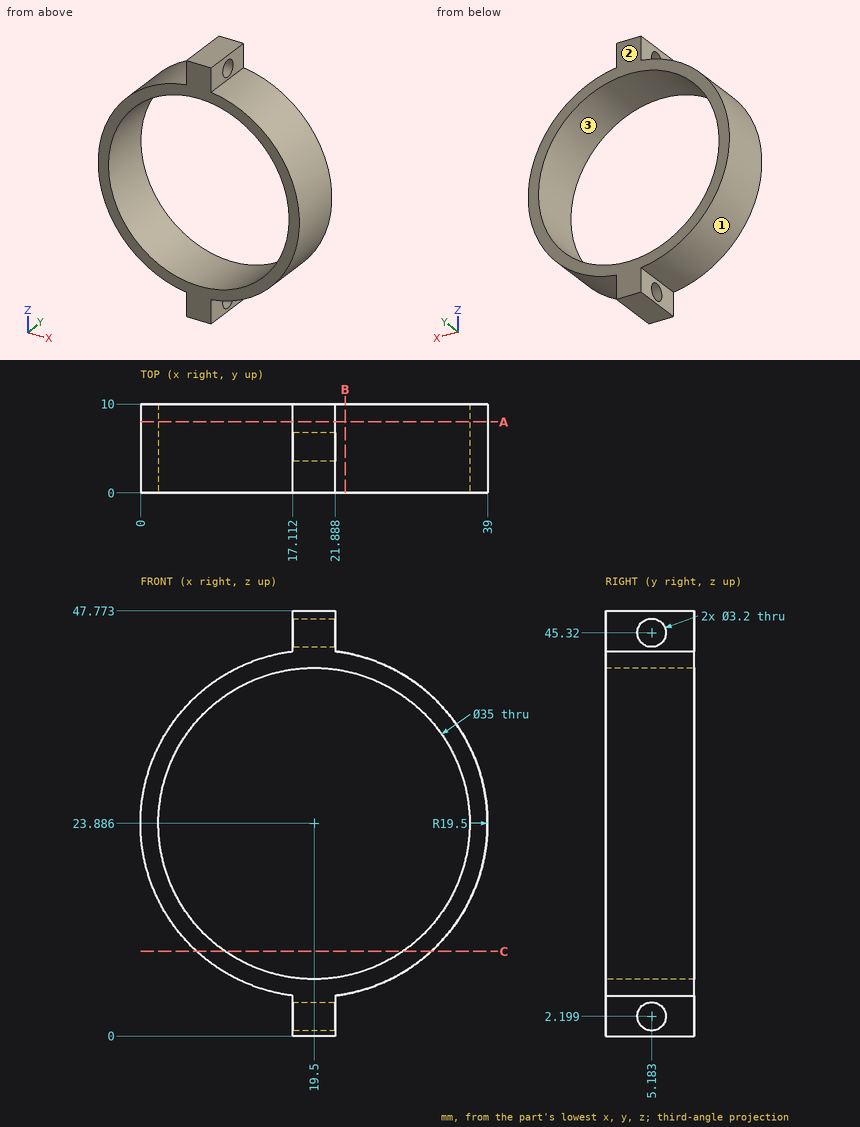
For this review, use the dimensioned drawing (mm, ordinates from the lowest corner) and the shaded views. Give positions to 0.01 mm unless a question says otherwise; leave off trailing zeros. Order: outer loops, then holes, each group sorted by start corner. A loop starts at its lowest first (then second) coordinate and runs counter-clockwise, first axis right, second up. Notation, with made-up numbers: (-21, 42) - (13, 42) arc R21 ccw to (13, 78) - close; hole circle Ø9 at (47, 65). An arc over 180 degrees is marked (long way). Write item = value, one per line. Start each with the question number.
Q1. We need section B-B on x = 23. State the section outline as (y, z) points.
Q2. Clearance check with flat-ended pins moving along their axes: pin 1 Ø1 at (y, z) = (1.5, 12.5) entering from +X; pin 2 Ø2.5 at (y, z) = (3.5, 45) entering from -X; pin 3 Ø1 at (y, z) = (1.5, 27) entering from +X; pin 4 Ø21 at (x, z) = (19.5, 23.89) entering from -Y. State where each tip first meets the part, or that it passes through.
Q3. To check wall thickness, follow L1, parallel to X at y = 6, z = 13; L2, parallel to Z at x = 10.5, y = 8.75 (1 decimal); L3, parallel to X at y = 1.5, z = 15.5 (1 decimal). State the ranges of each line that lie inside material, in increasing order. Write a range as from..to.
Q4. We need section A-A on y = 8. State the section outline as (x, z) points.
Q5. We need section C-C on z = 9.5. State the section outline as (x, y) points.
Q6. Mouldability with a two-part tool opening along X and no side actions: class the marked faces 1, 2 and 3 as released by +X, released by -X, zero draft, split by the parting line, or undercut.
Working result:
q1.outline = (0, 4.7) - (10, 4.7) - (10, 6.74) - (0, 6.74) - close; (0, 41.03) - (10, 41.03) - (10, 43.07) - (0, 43.07) - close
q2.pin_1 = 35.68
q2.pin_2 = 17.11
q2.pin_3 = 38.82
q2.pin_4 = through
q3.L1 = 3.32..5.8, 33.2..35.68
q3.L2 = 6.6..8.9, 38.9..41.2
q3.L3 = 1.9..4.1, 34.9..37.1
q4.outline = (17.11, 0) - (21.89, 0) - (21.89, 4.53) arc R19.5 ccw to (21.89, 43.24) - (21.89, 47.77) - (17.11, 47.77) - (17.11, 43.24) arc R19.5 ccw to (17.11, 4.53) - close; hole circle Ø35 at (19.5, 23.89)
q5.outline = (6.34, 0) - (9.54, 0) - (9.54, 10) - (6.34, 10) - close; (29.46, 0) - (32.66, 0) - (32.66, 10) - (29.46, 10) - close
q6.face_1 = released by -X
q6.face_2 = zero draft
q6.face_3 = undercut
